For this review, take the finished solid that the model builds, in its own axes (mm). Give positions to 0.01 mm unless a question says otherwise; leave off trailing zeros. Order: outer loops, then holes, each group sorted by start corner. A loop starts at its lowest first (then second) coordinate and runs counter-clockwise, first axis right, second up. Notation, with made-up numbers: (-19, -32.75) -> (36, -32.75) arc R9 ccw to (36, -15.75) -> close; hole circle Ø9 at (58, -38). An arc over 180 degrees is marked (long way). One line per item, written item: value. Start each with the question number.
from build123d import *

# Parameters (mm, degrees)
SKETCH1_W           = 11
SKETCH1_H           = 40
BOSS_EXTRUDE1_DEPTH = 20
SKETCH2_W           = 10
SKETCH2_H           = 1
CUT_EXTRUDE2_DEPTH  = 40


with BuildPart() as part:
    # Sketch1 → Boss-Extrude1 (new, symmetric)
    with BuildSketch(Plane.XY):
        Rectangle(SKETCH1_W, SKETCH1_H)
    extrude(amount=BOSS_EXTRUDE1_DEPTH, both=True)

    # Sketch2 → Cut-Extrude2 (cut)
    with BuildSketch(Plane.XY.offset(20)):
        with Locations((-0.5, 18.5)):
            Rectangle(SKETCH2_W, SKETCH2_H)
        with Locations((-0.5, 17.250002203)):
            Rectangle(SKETCH2_W, SKETCH2_H)
        with Locations((-0.5, 16.000004405)):
            Rectangle(SKETCH2_W, SKETCH2_H)
        with Locations((-0.5, 14.750006608)):
            Rectangle(SKETCH2_W, SKETCH2_H)
        with Locations((-0.5, 13.50000881)):
            Rectangle(SKETCH2_W, SKETCH2_H)
        with Locations((-0.5, 12.250011013)):
            Rectangle(SKETCH2_W, SKETCH2_H)
        with Locations((-0.5, 11.000013216)):
            Rectangle(SKETCH2_W, SKETCH2_H)
        with Locations((-0.5, 9.750015418)):
            Rectangle(SKETCH2_W, SKETCH2_H)
        with Locations((-0.5, 8.500017621)):
            Rectangle(SKETCH2_W, SKETCH2_H)
        with Locations((-0.5, 7.250019823)):
            Rectangle(SKETCH2_W, SKETCH2_H)
        with Locations((-0.5, 6.000022026)):
            Rectangle(SKETCH2_W, SKETCH2_H)
        with Locations((-0.5, 4.750024229)):
            Rectangle(SKETCH2_W, SKETCH2_H)
        with Locations((-0.5, 3.500026431)):
            Rectangle(SKETCH2_W, SKETCH2_H)
        with Locations((-0.5, 2.250028634)):
            Rectangle(SKETCH2_W, SKETCH2_H)
        with Locations((-0.5, 1.000030836)):
            Rectangle(SKETCH2_W, SKETCH2_H)
        with Locations((-0.5, -0.249966961)):
            Rectangle(SKETCH2_W, SKETCH2_H)
        with Locations((-0.5, -1.499964758)):
            Rectangle(SKETCH2_W, SKETCH2_H)
        with Locations((-0.5, -2.749962556)):
            Rectangle(SKETCH2_W, SKETCH2_H)
        with Locations((-0.5, -3.999960353)):
            Rectangle(SKETCH2_W, SKETCH2_H)
        with Locations((-0.5, -5.249958151)):
            Rectangle(SKETCH2_W, SKETCH2_H)
        with Locations((-0.5, -6.499955948)):
            Rectangle(SKETCH2_W, SKETCH2_H)
        with Locations((-0.5, -7.749953745)):
            Rectangle(SKETCH2_W, SKETCH2_H)
        with Locations((-0.5, -8.999951543)):
            Rectangle(SKETCH2_W, SKETCH2_H)
        with Locations((-0.5, -10.24994934)):
            Rectangle(SKETCH2_W, SKETCH2_H)
        with Locations((-0.5, -11.499947138)):
            Rectangle(SKETCH2_W, SKETCH2_H)
        with Locations((-0.5, -12.749944935)):
            Rectangle(SKETCH2_W, SKETCH2_H)
        with Locations((-0.5, -13.999942732)):
            Rectangle(SKETCH2_W, SKETCH2_H)
        with Locations((-0.5, -15.24994053)):
            Rectangle(SKETCH2_W, SKETCH2_H)
        with Locations((-0.5, -16.499938327)):
            Rectangle(SKETCH2_W, SKETCH2_H)
        with Locations((-0.5, -17.749936125)):
            Rectangle(SKETCH2_W, SKETCH2_H)
    extrude(amount=-CUT_EXTRUDE2_DEPTH, mode=Mode.SUBTRACT)


solid = part.part
Q1. For line 1 along X through (y, z) = (-7.5, -7), list the stretches that pass through material, from the lowest coordinate up.
Q2. Take a section at A-A (x = -1.75). State how many separate pieces and enclosed holes the cut face has, and give its area (3 significant figures).
Q3. Take a section at B-B (y = -4). State the section outline as (x, z) points, and give its area (3 significant figures).
Answers below:
1. line 1: x = 4.5 to 5.5
2. separate pieces: 31
2. enclosed holes: 0
2. area: 400 mm²
3. outline: (4.5, -20) -> (5.5, -20) -> (5.5, 20) -> (4.5, 20) -> close
3. area: 40.0 mm²
